Source: CAD feature listing. Evaluate the final solid. Frame: model axes, mm. A direction names the side the tool comes from. Round coordinates to 2 decimals unless told otherwise and drop trailing zeros. Loops run counter-clockwise (first coordinate to the right, second up) from the corner with the lowest first, then second, coordinate; pieces in that order, holes last. Notation, with made-up numbers: (8, 1) -> (58, 1) arc R36 ccw to (58, 35) -> close; hole circle Ø8 at (27, -34.75). An arc over 180 degrees is marked (long way). Return JSON: item names as keys, results as strings. Group by question number.
```python
from build123d import *

# Parameters (mm, degrees)
BOSS_EXTRUDE2_DEPTH = 101.6
FILLET3_R           = 1
FILLET5_R           = 5
SKETCH8_R           = 3.175
CUT_EXTRUDE3_DEPTH  = 19.05
SKETCH9_W           = 19.05
SKETCH9_H           = 19.05
CUT_EXTRUDE4_DEPTH  = 12.7
FILLET6_R           = 5.08
SKETCH11_W          = 8
SKETCH11_H          = 12
CUT_EXTRUDE5_DEPTH  = 12.7
FILLET7_R           = 2.54


with BuildPart() as part:
    # Sketch2 → Boss-Extrude2 (new body)
    with BuildSketch(Plane(origin=(0, 0, 0), x_dir=(1, 0, 0), z_dir=(0, 1, 0))):
        with BuildLine():
            Line((-21.540573528, -21.56464913), (-28.275068663, -21.56464913))
            ThreePointArc((-28.275068663, -21.56464913), (-35.56, 0), (-28.275068663, 21.56464913))
            Line((-28.275068663, 21.56464913), (-21.540573528, 21.56464913))
            ThreePointArc((-21.540573528, 21.56464913), (-26.716830431, 14.671106698), (-29.7559672, 6.604))
            Line((-29.7559672, 6.604), (29.7559672, 6.604))
            ThreePointArc((29.7559672, 6.604), (26.716830431, 14.671106698), (21.540573528, 21.56464913))
            Line((21.540573528, 21.56464913), (28.275068663, 21.56464913))
            ThreePointArc((28.275068663, 21.56464913), (35.56, 0), (28.275068663, -21.56464913))
            Line((28.275068663, -21.56464913), (21.540573528, -21.56464913))
            ThreePointArc((21.540573528, -21.56464913), (26.840862889, -14.442938737), (29.864178944, -6.096))
            Line((29.864178944, -6.096), (-29.864178944, -6.096))
            ThreePointArc((-29.864178944, -6.096), (-26.840862889, -14.442938737), (-21.540573528, -21.56464913))
        make_face()
    extrude(amount=BOSS_EXTRUDE2_DEPTH)

    # Fillet3
    fillet3_edges = [part.edges().sort_by_distance(p)[0] for p in [
        (21.540573528, 50.8, -21.56464913),
        (28.275068663, 50.8, -21.56464913),
        (28.275068663, 50.8, 21.56464913),
        (21.540573528, 50.8, 21.56464913),
        (-21.540573528, 50.8, 21.56464913),
        (-28.275068663, 50.8, 21.56464913),
        (-28.275068663, 50.8, -21.56464913),
        (-21.540573528, 50.8, -21.56464913),
    ]]
    fillet(fillet3_edges, radius=FILLET3_R)

    # Fillet5
    fillet5_edges = [part.edges().sort_by_distance(p)[0] for p in [
        (29.864178944, 50.8, 6.096),
        (-29.864178944, 50.8, 6.096),
        (-29.7559672, 50.8, -6.604),
        (29.7559672, 50.8, -6.604),
    ]]
    fillet(fillet5_edges, radius=FILLET5_R)

    # Sketch8 → Cut-Extrude3 (cut)
    with BuildSketch(Plane(origin=(0, 101.6, 0), x_dir=(1, 0, 0), z_dir=(0, 1, 0))):
        Circle(SKETCH8_R)
    extrude(amount=-CUT_EXTRUDE3_DEPTH, mode=Mode.SUBTRACT)

    # Sketch9 → Cut-Extrude4 (cut)
    with BuildSketch(Plane.XY.offset(6.096)):
        with Locations((-0.285711728, 92.075)):
            Rectangle(SKETCH9_W, SKETCH9_H)
    extrude(amount=-CUT_EXTRUDE4_DEPTH, mode=Mode.SUBTRACT)

    # Fillet6
    fillet6_edges = [part.edges().sort_by_distance(p)[0] for p in [
        (9.239288272, 82.55, -0.254),
        (-9.810711728, 82.55, -0.254),
    ]]
    fillet(fillet6_edges, radius=FILLET6_R)

    # Sketch11 → Cut-Extrude5 (cut)
    with BuildSketch(Plane.XY.offset(6.096)):
        with Locations((12.587070083, 0)):
            Rectangle(SKETCH11_W, SKETCH11_H)
    extrude(amount=-CUT_EXTRUDE5_DEPTH, mode=Mode.SUBTRACT)

    # Fillet7
    fillet7_edges = [part.edges().sort_by_distance(p)[0] for p in [
        (16.587070083, 6, -0.254),
        (8.587070083, 6, -0.254),
    ]]
    fillet(fillet7_edges, radius=FILLET7_R)


solid = part.part
```
(1) Pin query (flat end, axial travel): pin 1 (1 mm diameter, centred on y = 2, z = 0.5, fed in from -X); pin 2 (1 mm diameter, centred on x = 16, y = 67.5, fed in from -Z); pin 3 (0.9 mm diameter, centred on x = 12.5, z = 0, fed in from -Y); pin 4 (10 mm diameter, centred on x = 20, y = 61.5, fed in from -Z). Return the tip coordinate at first contact, or that it passes through.
(2) Ray query, line 1 (Z direction, x = 24, y = 16); line 2 (X direction, y = 58, z = 1); line 3 (X direction, y = 43, z = -14). Return the intervals inside material, ascending.
(3) Cut plane D-D (x = -3). Return loops of the section in (y, z).
(4) Cut plane A-A (y = 28). Return loops of the section in (x, z), and give its area (3 significant figures).
(5) Mould query, pull axis X, two halves, no side actions, for faces 4 (the face through (35.56, 50.09, -0.32)), 5 (the face through (27.135, 51.511, 8.38)), 6 (the face through (-26, 50, 21.565)). Classes: released by +X, released by -X, zero draft, split by the parting line, or undercut.
(6) Cut plane B-B (z = -18.5). Return loops of the section in (x, y).
(7) Set-up query: faces 1 (the face through (-9.811, 95, 0)), 2 (the face through (26.91, 51.51, -8.93)), 3 (the face through (0, 50, -6.604)). Return all of +Z, -Z, +X, -X, +Y, -Y with unobstructed straight access to the full face (end or side cutting, diameter ignored); none if empty.
(8) Cut plane C-C (z = 0). Return loops of the section in (x, y), and give its area (3 significant figures).
Answers follow:
{
 "1": {"pin 1": "x = -35.56", "pin 2": "z = -6.6", "pin 3": "y = 6", "pin 4": "z = -21.56"},
 "2": {"line 1": "-21.56 to -18.79, -6.78 to 6.21, 18.79 to 21.56", "line 2": "-35.55 to 35.55", "line 3": "-32.69 to -27.07, 27.07 to 32.69"},
 "3": {"outline": "(0, -6.6) -> (82.55, -6.6) -> (82.55, 6.1) -> (0, 6.1) -> close"},
 "4": {"outline": "(-28.58, -21.16) arc R1 ccw to (-27.78, -21.56) -> (-23.83, -21.56) arc R1 ccw to (-23.08, -19.91) arc R30.48 cw to (-27.14, -13.88) arc R5 cw to (-22.68, -6.6) -> (22.68, -6.6) arc R5 cw to (27.14, -13.88) arc R30.48 cw to (23.08, -19.91) arc R1 ccw to (23.83, -21.56) -> (27.78, -21.56) arc R1 ccw to (28.58, -21.16) arc R35.56 ccw to (28.58, 21.16) arc R1 ccw to (27.78, 21.56) -> (23.83, 21.56) arc R1 ccw to (23.08, 19.91) arc R30.48 cw to (27.44, 13.27) arc R5 cw to (22.94, 6.1) -> (-22.94, 6.1) arc R5 cw to (-27.44, 13.27) arc R30.48 cw to (-23.08, 19.91) arc R1 ccw to (-23.83, 21.56) -> (-27.78, 21.56) arc R1 ccw to (-28.58, 21.16) arc R35.56 ccw to start", "area": "1,290 mm^2"},
 "5": {"face 4": "released by +X", "face 5": "undercut", "face 6": "zero draft"},
 "6": {"outline": "(-30.37, 0) -> (-24.22, 0) -> (-24.22, 101.6) -> (-30.37, 101.6) -> close; (24.22, 0) -> (30.37, 0) -> (30.37, 101.6) -> (24.22, 101.6) -> close"},
 "7": {"face 1": "+Z, -Z, +Y", "face 2": "+Y, -Y", "face 3": "-Z, +Y, -Y"},
 "8": {"outline": "(-35.56, 0) -> (8.59, 0) -> (8.59, 3.46) arc R2.54 cw to (11.13, 6) -> (14.05, 6) arc R2.54 cw to (16.59, 3.46) -> (16.59, 0) -> (35.56, 0) -> (35.56, 101.6) -> (9.24, 101.6) -> (9.24, 87.63) arc R5.08 cw to (4.16, 82.55) -> (-4.73, 82.55) arc R5.08 cw to (-9.81, 87.63) -> (-9.81, 101.6) -> (-35.56, 101.6) -> close", "area": "6,830 mm^2"}
}
